The drawing under review shows one solid part. Ordinate dimensions are in mm from its lowest x, y, z. Coordinates: 2 decimals unless noted, no trailing zeros. Write each loop counter-clockwise with the first axis right and the second up, starting at its lowest first coordinate (ties: lowest second). Pieces come first, ordered by that corner, then holes. Notation, with made-up numbers: (-29.5, 2.25) - (9.5, 2.25) arc R11 cw to (9.5, 21.25) - close; hole circle Ø4 at (60.5, 16). An arc over 180 degrees is marked (long way). Use a Markdown table: item, result.
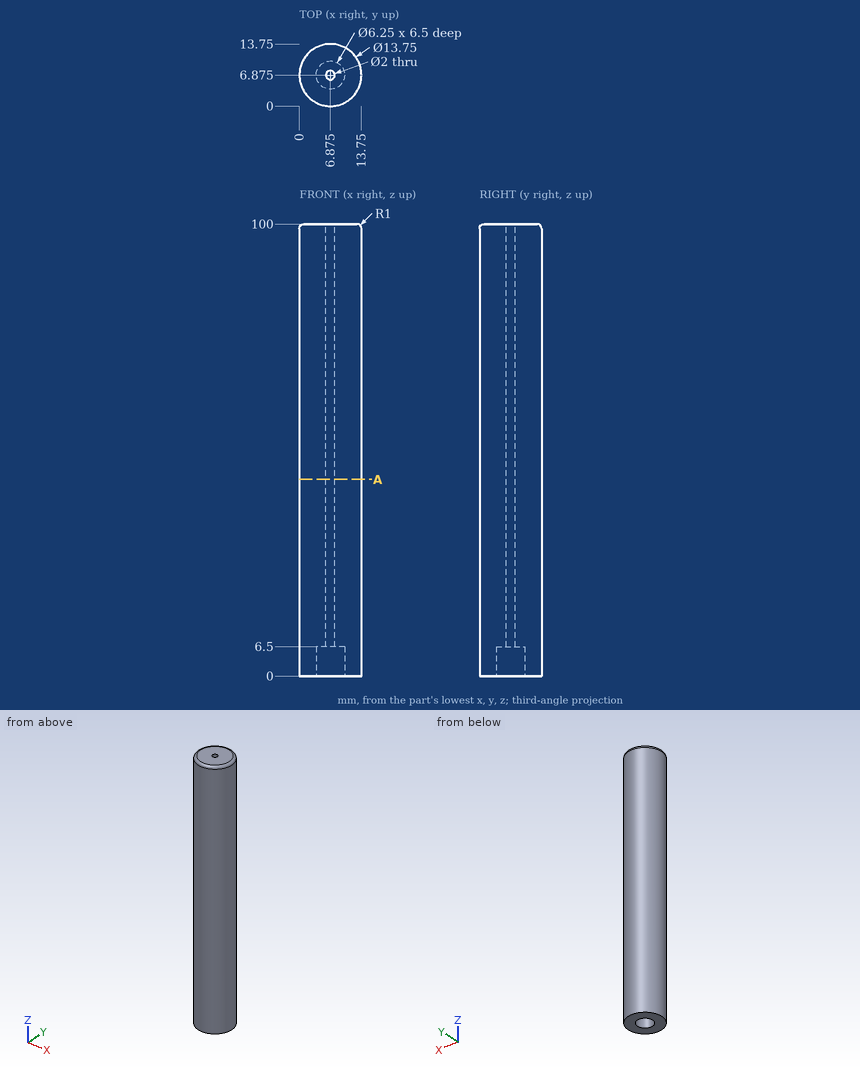
(1) For pin 1 (3 mm diameter, centred on x = 6.875, y = 6.875, fed in from -Z); pin 2 (1 mm diameter, centred on y = 9.5, z = 36, fed in from +X); pin 3 (3 mm diameter, centred on x = 4.5, z = 70.5, fed in from -Y), all flat-tipped, find the tip position at first contact; note any pin that passes through.
Determined:
| item | result |
|---|---|
| pin 1 | z = 6.5 |
| pin 2 | x = 13.41 |
| pin 3 | y = 0.06 |
(2) Take a section at A-A on z = 43.5. Write out the cut boundary in (x, y) (3 decimals), and give its area (3 significant figures).
Determined:
| item | result |
|---|---|
| outline | circle Ø13.75 at (6.875, 6.875); hole circle Ø2 at (6.875, 6.875) |
| area | 145 mm2 |
(3) For L1, parallel to Y at x = 7, z = 49; L2, parallel to Z at x = 7, y = 9; L3, parallel to X at y = 7.5, z = 69, list the stretches that pass through material, from the lowest coordinate up. Write a range as from..to.
Determined:
| item | result |
|---|---|
| L1 | 0..5.88, 7.87..13.75 |
| L2 | 6.5..100 |
| L3 | 0.03..6.09, 7.66..13.72 |
